Verification items for this drawing (mm, ordinates from the low corner). A direction names the side the tool comes from. Round coordinates to 2 decimals unless told otherwise and drop trailing zeros. Order: outer loops, then holes, each group sorted by start corner. A loop starts at its lowest first (then second) coordinate and runs counter-clockwise, first axis right, second up. Notation, with made-up numbers: (56.25, -32) - (92.25, -32) arc R23 ccw to (92.25, 0) - close; hole circle Ø3 at (4, 30). An arc over 180 degrees is marked (long way). Use a Markdown table: item, result. Add a question column.
(1) Mould release check, pull along X, two halves, no side actions. Record for the marked faces 1, 2 and 3: released by +X, released by -X, zero draft, split by the parting line, or undercut.
(2) Section check D-D on z = 14. Record the boundary of the cut face in (x, y).
(3) Section check A-A on y = 16. Record the boundary of the cut face in (x, z).
(4) Section check B-B on x = 28. Record the boundary of the cut face in (y, z), then the cut area to 3 significant figures.
(5) Gauge pin test, flat ends, axial feed: P1, Ø7, axis at x = 18.5, y = 20, coming from the -Z side; P2, Ø11, axis at x = 15, z = 44, coming from the +Y side. Record the tip position at first contact, or that the pin passes through.
(6) Access from +Z, -Z, +X, -X, +Y, -Y to the whole of each face (thin tool, end or side, straight path). Record for the marked faces 4 and 5.
(7) Thickness scan on line 1 along X through (y, z) = (20.75, 50); line 2 along Y through (x, z) = (29.5, 56.5); line 3 along Y through (x, z) = (14, 6.5). Record the ranges inside material, lowest first. Write a range as [from, to].
(8) Section check C-C on z = 52.5. Record the boundary of the cut face in (x, y).
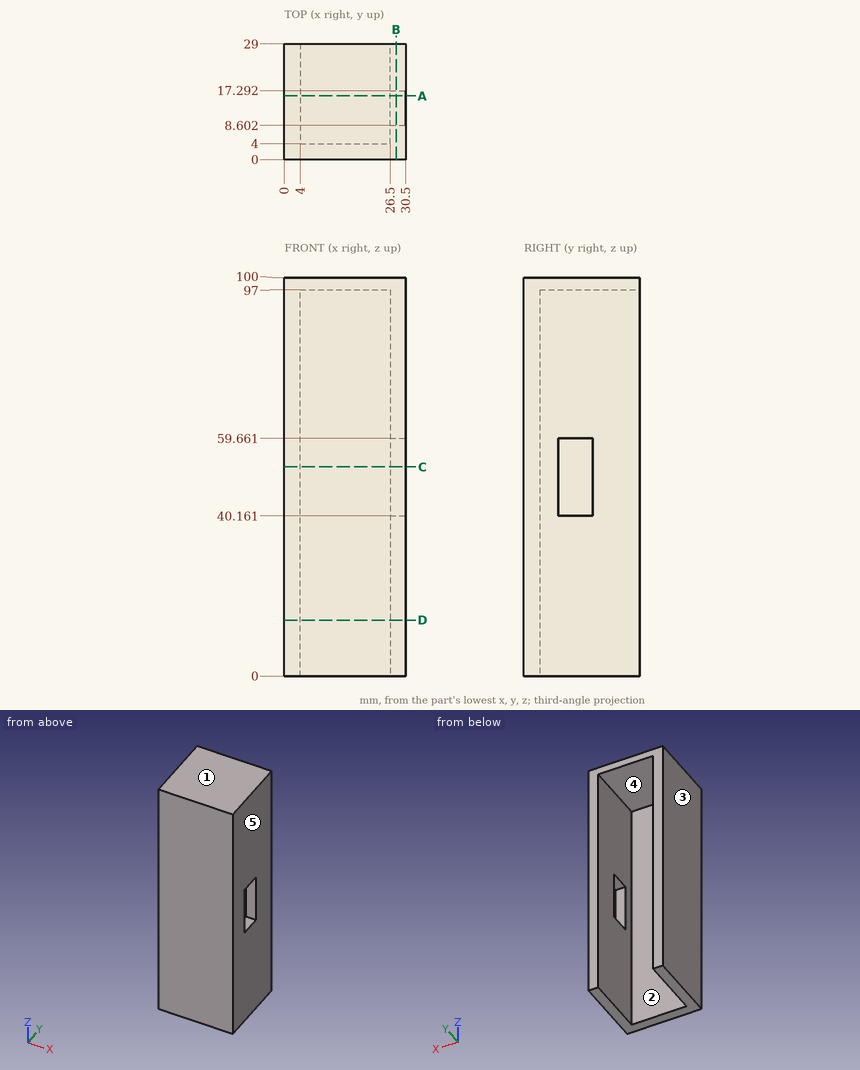
Check sheet entries:
| question | item | result |
|---|---|---|
| 1 | face 1 | zero draft |
| 1 | face 2 | undercut |
| 1 | face 3 | released by -X |
| 2 | outline | (0, 0) - (30.5, 0) - (30.5, 29) - (26.5, 29) - (26.5, 4) - (4, 4) - (4, 29) - (0, 29) - close |
| 3 | outline | (0, 0) - (4, 0) - (4, 97) - (26.5, 97) - (26.5, 59.66) - (30.5, 59.66) - (30.5, 100) - (0, 100) - close; (26.5, 0) - (30.5, 0) - (30.5, 40.16) - (26.5, 40.16) - close |
| 4 | outline | (0, 0) - (29, 0) - (29, 100) - (0, 100) - close; hole (8.6, 40.16) - (17.29, 40.16) - (17.29, 59.66) - (8.6, 59.66) - close |
| 4 | area | 2,730 mm2 |
| 5 | P1 | stops at z = 97 |
| 5 | P2 | stops at y = 4 |
| 6 | face 4 | -Z, +Y |
| 6 | face 5 | +Z, -Z, +X, +Y, -Y |
| 7 | line 1 | x = [0, 4], [26.5, 30.5] |
| 7 | line 2 | y = [0, 8.6], [17.29, 29] |
| 7 | line 3 | y = [0, 4] |
| 8 | outline | (0, 0) - (30.5, 0) - (30.5, 8.6) - (26.5, 8.6) - (26.5, 4) - (4, 4) - (4, 29) - (0, 29) - close; (26.5, 17.29) - (30.5, 17.29) - (30.5, 29) - (26.5, 29) - close |
